Build history of the part. All positions in model axes, mm. A direction names the side the tool comes from. Round coordinates to 2 decimals unless told otherwise and drop trailing zeros. Loops run counter-clockwise (first coordinate to the right, second up) from the corner with the lowest first, then second, coordinate; pieces in that order, holes last. Notation, with made-up numbers: (-36, 79.25) - (6, 79.25) arc R12 cw to (6, 96.25) - close; hole circle Ø2 at (53.5, -35.75). An arc over 180 degrees is marked (long way). Put each result on its own line as item: value. Start each with the question number.
from build123d import *

# Parameters (mm, degrees)
SKETCH_1_W          = 41.3
SKETCH_1_H          = 28.5
EXTRUDE_1_DEPTH     = 1.2
SKETCH_2_R          = 3.466188446
EXTRUDE_2_DEPTH     = 9.5
SKETCH_3_W          = 7.4
SKETCH_3_H          = 5.8
EXTRUDE_3_DEPTH     = 7.1
HOLE_WIZARD_M2_1_D  = 2.6
SKETCH_6_W          = 0.968388925
SKETCH_6_H          = 8.634886507
EXTRUDE_4_DEPTH     = 4
SKETCH_7_W          = 6.634886507
SKETCH_7_H          = 3
CUT_EXTRUDE_1_DEPTH = 35.282372501
EXTRUDE_START       = -9.5
SKETCH_8_W          = 6.932376893
SKETCH_8_H          = 6.932376892
EXTRUDE_5_DEPTH     = 8.5
SKETCH_9_R          = 1.463933671
SKETCH_9_R_2        = 0.77068749
EXTRUDE_6_DEPTH     = 6
EXTRUDE_7_DEPTH     = 2
EXTRUDE_START_2     = -1.5
SKETCH_11_W         = 2
SKETCH_11_H         = 2
EXTRUDE_8_DEPTH     = 2.5
SKETCH_12_W         = 9.968388925
SKETCH_12_H         = 0.413345803
CUT_EXTRUDE_3_DEPTH = 1.5


with BuildPart() as part:
    # 草图1 → 凸台-拉伸1 (new body)
    with BuildSketch(Plane(origin=(0, 0, 0), x_dir=(1, 0, 0), z_dir=(0, 1, 0))):
        Rectangle(SKETCH_1_W, SKETCH_1_H)
    extrude(amount=EXTRUDE_1_DEPTH)

    # 草图2 → 凸台-拉伸2 (add)
    with BuildSketch(Plane(origin=(0, 1.2, 0), x_dir=(1, 0, 0), z_dir=(0, 1, 0))):
        with Locations(Location((-14.151249329, 5.368489825, 0), (0, 0, 270))):
            Circle(SKETCH_2_R)
    extrude(amount=EXTRUDE_2_DEPTH)

    # 草图3 → 凸台-拉伸3 (add)
    with BuildSketch(Plane.XZ):
        Rectangle(SKETCH_3_W, SKETCH_3_H)
    extrude(amount=EXTRUDE_3_DEPTH)

    # M2 间隙孔1 (through all)
    with Locations(Plane(origin=(0, 0, 0), x_dir=(-1, 0, 0), z_dir=(0, -1, 0))):
        with Locations((18, -12), (-18, -12), (-18, 12), (18, 12)):
            Hole(HOLE_WIZARD_M2_1_D / 2)

    # 草图6 → 凸台-拉伸4 (add)
    with BuildSketch(Plane(origin=(0, 1.2, 0), x_dir=(1, 0, 0), z_dir=(0, 1, 0))):
        with Locations((-4.46731767, -15.732556747)):
            Rectangle(SKETCH_6_W, SKETCH_6_H)
        with Locations((-1.46731767, -15.732556747)):
            Rectangle(SKETCH_6_W, SKETCH_6_H)
        with Locations((1.53268233, -15.732556747)):
            Rectangle(SKETCH_6_W, SKETCH_6_H)
        with Locations((4.53268233, -15.732556747)):
            Rectangle(SKETCH_6_W, SKETCH_6_H)
    extrude(amount=EXTRUDE_4_DEPTH)

    # 草图7 → 切除-拉伸1 (cut, through all)
    with BuildSketch(Plane(origin=(5.016876792, 0, 0), x_dir=(0, 0, -1), z_dir=(1, 0, 0))):
        with Locations((-16.732556747, 2.7)):
            Rectangle(SKETCH_7_W, SKETCH_7_H)
    extrude(amount=-CUT_EXTRUDE_1_DEPTH, mode=Mode.SUBTRACT)

    # 草图8 → 凸台-拉伸5 (add)
    with BuildSketch(Plane(origin=(0, 10.7, 0), x_dir=(1, 0, 0), z_dir=(0, 1, 0)).offset(EXTRUDE_START)):
        with Locations((-14.15124933, 5.368489825)):
            Rectangle(SKETCH_8_W, SKETCH_8_H)
    extrude(amount=EXTRUDE_5_DEPTH)

    # 草图9 → 凸台-拉伸6 (add)
    with BuildSketch(Plane(origin=(0, 1.2, 0), x_dir=(1, 0, 0), z_dir=(0, 1, 0))):
        with Locations(Location((-14.229613701, -7.405223715, 0), (0, 0, 270))):
            Circle(SKETCH_9_R)
        with Locations(Location((-10.0444332, -7.405223715, 0), (0, 0, 270))):
            Circle(SKETCH_9_R_2)
    extrude(amount=EXTRUDE_6_DEPTH)

    # 草图10 → 凸台-拉伸7 (add)
    with BuildSketch(Plane(origin=(0, 1.2, 0), x_dir=(1, 0, 0), z_dir=(0, 1, 0))):
        with BuildLine():
            Line((14.081901448, -3.613942556), (14.081901448, -9.128533333))
            ThreePointArc((14.081901448, -9.128533333), (12.703253753, -10.507181027), (11.324606059, -9.128533333))
            Line((11.324606059, -9.128533333), (11.324606059, -3.613942556))
            ThreePointArc((11.324606059, -3.613942556), (12.703253753, -2.235294862), (14.081901448, -3.613942556))
        make_face()
    extrude(amount=EXTRUDE_7_DEPTH)

    # 草图11 → 凸台-拉伸8 (add)
    with BuildSketch(Plane(origin=(0, 5.2, 0), x_dir=(1, 0, 0), z_dir=(0, 1, 0)).offset(EXTRUDE_START_2)):
        with Locations((-4.46731767, -12.415113493)):
            Rectangle(SKETCH_11_W, SKETCH_11_H)
        with Locations((-1.46731767, -12.415113493)):
            Rectangle(SKETCH_11_W, SKETCH_11_H)
        with Locations((4.53268233, -12.415113493)):
            Rectangle(SKETCH_11_W, SKETCH_11_H)
        with Locations((1.53268233, -12.415113493)):
            Rectangle(SKETCH_11_W, SKETCH_11_H)
    extrude(amount=-EXTRUDE_8_DEPTH)

    # 草图12 → 切除-拉伸3 (cut)
    with BuildSketch(Plane(origin=(0, 5.2, 0), x_dir=(1, 0, 0), z_dir=(0, 1, 0))):
        with Locations((0.03268233, -11.621786395)):
            Rectangle(SKETCH_12_W, SKETCH_12_H)
    extrude(amount=-CUT_EXTRUDE_3_DEPTH, mode=Mode.SUBTRACT)


solid = part.part
Item 1: Which spindle directions (+Z, -Z, +X, -X, +Y, -Y) get a long thin tool onto all of the face, cutting with end or side? Do faces 4 (the flat face through (-5.467, 2, 12)), 5 (the flat face through (-4, 3, 13.415)), 6 (the flat face through (1.5, 4.5, 11.828)), 7 (the flat face through (5.017, 5, 16)). Say none if no direction does.
Item 2: Drill centre lines: probe 1 along Z at (x, y) = (18, 0.85); probe 2 along X at (y, z) = (0.3, 12); probe 3 along Y at (x, z) = (1.5, -2.5). Where is each one in solid material? Low to high. Write a range as [from, to].
Item 3: Slice it at D-D (y = 2.25). Give the cut face in (x, z), plus the area to 3 significant figures.
Item 4: Slice it at A-A (z = -11.5). Give the cut face in (x, y).
Item 5: Slice it at B-B (x = 18). Give the cut face in (y, z), plus the area to 3 significant figures.
Item 6: Slice it at C-C (z = 16). Give the cut face in (x, y).
Item 7: Drop flat-ended pins along their axis: pin 1 Ø3 at (x, y) = (12.5, 3.5) entering from -Z; pin 2 Ø4 at (x, y) = (-9.5, 7) entering from +Z; pin 3 Ø2 at (x, y) = (-1.5, -5.5) entering from -Z. Give the stop position or say it passes through.
Item 8: Two-plate mould, pull along X, no slides. Class faces 1 (the flat face through (-17, 9.7, -3)), 2 (the flat face through (11.325, 2, 6)), 3 (the cylindrical face through (12.673, 2.186, 2.236)): pulls with the +X half, pulls with the -X half, needs draft (parallel to the pull), parting line crosses it, or undercut.
Computed values:
1. face 4: +Z, -Z, -X, +Y
1. face 5: +Z, +X, -X
1. face 6: -Z, +X, -X, +Y
1. face 7: +Z, -Z, +X, +Y
2. probe 1: z = [-14.25, -13.3], [-10.7, 10.7], [13.3, 14.25]
2. probe 2: x = [-20.65, -19.3], [-16.7, 16.7], [19.3, 20.65]
2. probe 3: y = [-7.1, 1.2]
3. outline: (-17.62, -8.83) - (-10.69, -8.83) - (-10.69, -1.9) - (-17.62, -1.9) - close; circle Ø2.93 at (-14.23, 7.41); circle Ø1.54 at (-10.04, 7.41); (-5.47, 11.42) - (-3.47, 11.42) - (-3.47, 13.42) - (-5.47, 13.42) - close; (-2.47, 11.42) - (-0.47, 11.42) - (-0.47, 13.42) - (-2.47, 13.42) - close; (0.53, 11.42) - (2.53, 11.42) - (2.53, 13.42) - (0.53, 13.42) - close; (3.53, 11.42) - (5.53, 11.42) - (5.53, 13.42) - (3.53, 13.42) - close; (11.32, 3.61) arc R1.38 ccw to (14.08, 3.61) - (14.08, 9.13) arc R1.38 ccw to (11.32, 9.13) - close
3. area: 93.8 mm^2
4. outline: (-20.65, 0) - (-19.2, 0) - (-19.2, 1.2) - (-20.65, 1.2) - close; (-16.8, 0) - (16.8, 0) - (16.8, 1.2) - (-16.8, 1.2) - close; (19.2, 0) - (20.65, 0) - (20.65, 1.2) - (19.2, 1.2) - close
5. outline: (0, -14.25) - (1.2, -14.25) - (1.2, -13.3) - (0, -13.3) - close; (0, -10.7) - (1.2, -10.7) - (1.2, 10.7) - (0, 10.7) - close; (0, 13.3) - (1.2, 13.3) - (1.2, 14.25) - (0, 14.25) - close
5. area: 28.0 mm^2
6. outline: (-4.95, 4.2) - (-3.98, 4.2) - (-3.98, 5.2) - (-4.95, 5.2) - close; (-1.95, 4.2) - (-0.98, 4.2) - (-0.98, 5.2) - (-1.95, 5.2) - close; (1.05, 4.2) - (2.02, 4.2) - (2.02, 5.2) - (1.05, 5.2) - close; (4.05, 4.2) - (5.02, 4.2) - (5.02, 5.2) - (4.05, 5.2) - close
7. pin 1: stops at z = 2.24
7. pin 2: stops at z = 8.18
7. pin 3: stops at z = -2.9
8. face 1: needs draft
8. face 2: undercut
8. face 3: parting line crosses it
